Model file for the job. Use its own axes, mm. Face numbers are marked on the shaded views. A direction names the side the tool comes from. Round coordinates to 2 decimals unless told otherwise and drop trailing zeros. Write each loop counter-clockwise with the first axis right and the second up, starting at its lowest first coordinate (ties: lowest second). Pieces come first, ordered by that corner, then holes.
```python
from build123d import *

# Parameters (mm, degrees)
SKETCH_1_W          = 40
SKETCH_1_H          = 20
EXTRUDE_1_DEPTH     = 4
SKETCH_2_R          = 6
EXTRUDE_2_DEPTH     = 5
SKETCH_3_W          = 40
SKETCH_3_H          = 35
CUT_EXTRUDE_1_DEPTH = 1
SKETCH_6_R          = 2.05
CUT_EXTRUDE_3_DEPTH = 10


with BuildPart() as part:
    # 草图1 → 凸台-拉伸1 (new body)
    with BuildSketch(Plane(origin=(0, 0, 0), x_dir=(1, 0, 0), z_dir=(0, 1, 0))):
        Rectangle(SKETCH_1_W, SKETCH_1_H)
    extrude(amount=-EXTRUDE_1_DEPTH)

    # 草图2 → 凸台-拉伸2 (add)
    with BuildSketch(Plane.XY.offset(10)):
        with BuildLine():
            Line((20, -4), (20, 0))
            Line((20, 0), (-20, 0))
            Line((-20, 0), (-20, -4))
            Line((-20, -4), (-8.121724647, -28.877832997))
            ThreePointArc((-8.121724647, -28.877832997), (0, -34), (8.121724647, -28.877832997))
            Line((8.121724647, -28.877832997), (20, -4))
        make_face()
        with Locations((0, -25)):
            Circle(SKETCH_2_R, mode=Mode.SUBTRACT)
    extrude_2 = extrude(amount=EXTRUDE_2_DEPTH)

    # 草图3 → 切除-拉伸1 (cut)
    with BuildSketch(Plane(origin=(0, 0, 10), x_dir=(-1, 0, 0), z_dir=(0, 0, -1))):
        with Locations((0, -21.5)):
            Rectangle(SKETCH_3_W, SKETCH_3_H)
    cut_extrude_1 = extrude(amount=-CUT_EXTRUDE_1_DEPTH, mode=Mode.SUBTRACT)

    # 镜向1: 凸台-拉伸2, 切除-拉伸1 across plane
    add(extrude_2.mirror(Plane.XY))
    add(cut_extrude_1.mirror(Plane.XY), mode=Mode.SUBTRACT)

    # 草图6 → 切除-拉伸3 (cut)
    with BuildSketch(Plane.XZ.offset(4)):
        with Locations(Location((-10, 0, 0), (0, 0, 270))):
            Circle(SKETCH_6_R)
        with Locations(Location((10, 0, 0), (0, 0, 270))):
            Circle(SKETCH_6_R)
    extrude(amount=-CUT_EXTRUDE_3_DEPTH, mode=Mode.SUBTRACT)


solid = part.part
```
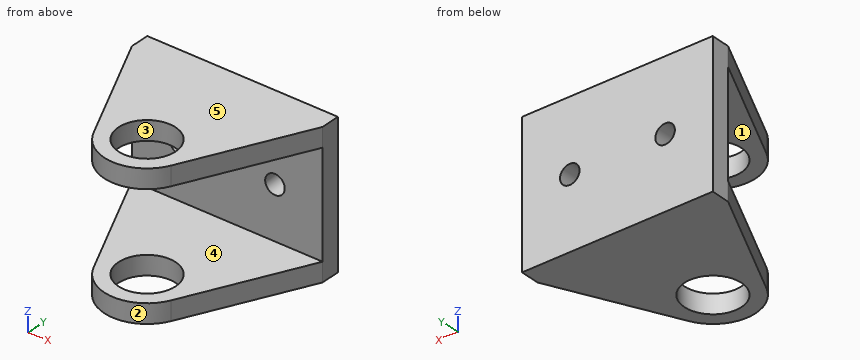
1) Cut at C-C on y = -12. List the corners of the cut face in (x, z), and give its area (3 significant figures).
2) Flat gauge pins, fed straight in: pin 1 Ø8 at (x, z) = (-0.5, -6.5) entering from +Y; pin 2 Ø6.5 at (x, z) = (10, 0) entering from -Y; pin 3 Ø4 at (y, z) = (-16.5, 10.5) entering from +X; pin 4 Ø9.5 at (x, y) = (0, -25) entering from -Z. Where does each tip first touch, or does it go through?
3) Which spindle directions (+Z, -Z, +X, -X, +Y, -Y) get a long thin tool onto all of the face, cutting with end or side? Do the marked faces 4 and 5. Say none if no direction does.
4) Cut at B-B on z = 0. List the corners of the cut face in (x, y), and give its area (3 significant figures).
5) Pull direction Y, two halves, no side cores. Call the marked faces 1, 2 and 3: released by +Y, released by -Y, zero draft, split by the parting line, or undercut.
6) Cut at A-A on x = 0. List the corners of the cut face in (y, z), and give its area (3 significant figures).
7) Wall check: probe 1 along Z at (x, y) = (-7, -25.5); probe 2 along Y at (x, z) = (0, 13.7); probe 3 along X at (y, z) = (-3, -1.75). Give the ranges that are in metal, low to high.
8) Cut at D-D on x = 10. List the corners of the cut face in (y, z).
Result sheet:
1. outline: (-16.18, -15) - (16.18, -15) - (16.18, -11) - (-16.18, -11) - close; (-16.18, 11) - (16.18, 11) - (16.18, 15) - (-16.18, 15) - close
1. area: 259 mm2
2. pin 1: stops at y = 0
2. pin 2: stops at y = -4
2. pin 3: stops at x = 14.96
2. pin 4: passes through
3. face 4: +X, -X, -Y
3. face 5: +Z, +X, -X, +Y, -Y
4. outline: (-20, -4) - (-12.05, -4) - (-12.05, 0) - (-20, 0) - close; (-7.95, -4) - (7.95, -4) - (7.95, 0) - (-7.95, 0) - close; (12.05, -4) - (20, -4) - (20, 0) - (12.05, 0) - close
4. area: 127 mm2
5. face 1: zero draft
5. face 2: released by -Y
5. face 3: undercut
6. outline: (-34, -15) - (-31, -15) - (-31, -11) - (-34, -11) - close; (-34, 11) - (-31, 11) - (-31, 15) - (-34, 15) - close; (-19, -15) - (0, -15) - (0, 15) - (-19, 15) - (-19, 11) - (-4, 11) - (-4, -11) - (-19, -11) - close
6. area: 264 mm2
7. probe 1: z = -15 to -11, 11 to 15
7. probe 2: y = -34 to -31, -19 to 0
7. probe 3: x = -20 to -11.07, -8.93 to 8.93, 11.07 to 20
8. outline: (-24.94, -15) - (0, -15) - (0, -2.05) - (-4, -2.05) - (-4, -11) - (-24.94, -11) - close; (-24.94, 11) - (-4, 11) - (-4, 2.05) - (0, 2.05) - (0, 15) - (-24.94, 15) - close
